Build history of the part. All positions in model axes, mm. Coordinates: 2 decimals unless noted, no trailing zeros. Write each loop counter-clockwise with the first axis right and the second up, starting at its lowest first coordinate (ties: lowest second). Pieces come first, ordered by that corner, then holes. Notation, with made-up numbers: (65.25, 6) -> (97.25, 6) arc R27 ccw to (97.25, 25) -> close; hole circle Ø6 at (23.25, 65). An arc over 180 degrees is marked (long way). Write each question's results on one line, items separated by ' | '. Start each with the question number.
Q1. Drill centre lines: line 1 (Y direction, x = 0, z = -11.5); line 2 (Y direction, x = 40.5, z = -87.5); line 3 (X direction, y = 489, z = -26). Where is each one in solid material? Low to high.
Q2. Saw through at A-A on z = -76. Give the cut face in (x, y).
Q3. Drop flat-ended pins along their axis: pin 1 Ø3 at (x, y) = (129.5, -433) entering from -Z; pin 2 Ø12 at (y, z) = (-133, -101) entering from +X; pin 3 Ø10 at (x, y) = (305.5, -282) entering from +Z. Give the stop position or say it passes through.
Q4. Two-plate mould, pull along X, no slides. Class faces 1 (the face through (78.108, 594.894, -15.21)), 2 (the face through (581, 136, 0)), 3 (the face through (-3.63, -16.35, -246.96)): released by +X, released by -X, zero draft, split by the parting line, or undercut.
Autodesk Inventor part; units mm, degrees
ref_plane "YZ Plane" through (0, 0, 0) normal (1, 0, 0) x (0, 1, 0)
ref_plane "XZ Plane" through (0, 0, 0) normal (0, 1, 0) x (-1, 0, 0)
ref_plane "XY Plane" through (0, 0, 0) normal (0, 0, 1) x (1, 0, 0)
sketch "Sketch1" plane through (0, 0, 0) normal (0, 1, 0) x (-1, 0, 0)
  line L0 (600, 0) -> (600, -30)
  arc A0 (541.7504, -124.6356) -> (600, -30) centre (494, -30) ccw
  arc A1 (15, -250) -> (541.7504, -124.6356) centre (15, 919.3202) ccw
  line L1 (0, 0) -> (0, -191.6842)
  arc A2 (15, -244) -> (539.0476, -119.2789) centre (15, 919.3202) ccw
  arc A3 (539.0476, -119.2789) -> (594, -30) centre (494, -30) ccw
  line L2 (594, -30) -> (594, 0)
  line L3 (594, 0) -> (600, 0)
  line L4 (0, -244) -> (0, -250)
  line L5 (0, -250) -> (15, -250)
  line L6 (0, -244) -> (15, -244)
  point P0 (0, 0)
  point P1 (0, -163.7009)
  point P2 (0, -169.7009)
  dimension "d1" = 30
  dimension "d3" = 1169.3202
  dimension "d11" = 1188
  dimension "d12" = 250
  dimension "d13" = 6
  dimension "d14" = 30
  dimension "d15" = 100
revolve "Revolution1" add sketch "Sketch1" angle 360 about axis through (0, 0, 0) along (0, 0, -1)
sketch "Sketch2" plane through (0, 0, 0) normal (0, 0, 1) x (1, 0, 0)
  circle A0 centre (0, 0) radius 16.75
  dimension "d8" = 33.5
extrude "Extrusion1" cut sketch "Sketch2" against normal through all
properties part number "PRS 1604 dished head D1000_1200"
Returned:
1) line 1: y = -600 to -594, 594 to 600 | line 2: y = -581.64 to -574.39, 574.39 to 581.64 | line 3: x = -347.68 to -337.22, 337.22 to 347.68
2) outline: circle Ø1179 at (0, 0); hole circle Ø1165.58 at (0, 0)
3) pin 1: stops at z = -165.9 | pin 2: stops at x = 562.42 | pin 3: stops at z = -170.94
4) face 1: split by the parting line | face 2: zero draft | face 3: undercut
